from build123d import *

# Parameters (mm, degrees)
SKETCH1_R           = 3.175
BOSS_EXTRUDE1_DEPTH = 1.3843


with BuildPart() as part:
    # Sketch1 → Boss-Extrude1 (new body, symmetric)
    with BuildSketch(Plane.XY):
        with BuildLine():
            Line((-9.281911907, 14.838161907), (-11.983546213, 3.110176509))
            ThreePointArc((-11.983546213, 3.110176509), (-11.495811318, 0.958331313), (-9.508369704, 0))
            Line((-9.508369704, 0), (9.508369704, 0))
            ThreePointArc((9.508369704, 0), (11.495811318, 0.958331313), (11.983546213, 3.110176509))
            Line((11.983546213, 3.110176509), (9.281911907, 14.838161907))
            ThreePointArc((9.281911907, 14.838161907), (0, 22.225), (-9.281911907, 14.838161907))
        make_face()
        with Locations((0, 12.7)):
            Circle(SKETCH1_R, mode=Mode.SUBTRACT)
    extrude(amount=BOSS_EXTRUDE1_DEPTH, both=True)


solid = part.part
Geometry check sheet. Reference: the model listing, model coordinates, mm. Round coordinates to 2 decimals unless told otherwise and drop trailing zeros. Order: outer loops, then holes, each group sorted by start corner. A loop starts at its lowest first (then second) coordinate and runs counter-clockwise, first axis right, second up. Notation, with made-up numbers: M 85,28 L 116,28 A33 cw 116,64 Z; hole C 9,2.5 d8. An arc over 180 degrees is marked long. Answer in a Markdown table with one row per item.
(1) Sectioned sample at A-A, the plane z = -0.9. Record the cut outline in (x, y) (3 decimals).
Responses:
| item | result |
|---|---|
| outline | M -11.984,3.11 A2.54 ccw -9.508,0 L 9.508,0 A2.54 ccw 11.984,3.11 L 9.282,14.838 A9.525 ccw -9.282,14.838 Z; hole C 0,12.7 d6.35 |
(2) Sectioned sample at D-D, the plane x = 5.5. Record the cut outline in (y, z), and give its area (3 significant figures).
Responses:
| item | result |
|---|---|
| outline | M 0,-1.38 L 20.48,-1.38 L 20.48,1.38 L 0,1.38 Z |
| area | 56.7 mm² |
(3) Sectioned sample at C-C, the plane y = 13.75. Record the cut outline in (x, z), and give its area (3 significant figures).
Responses:
| item | result |
|---|---|
| outline | M -9.53,-1.38 L -3,-1.38 L -3,1.38 L -9.53,1.38 Z; M 3,-1.38 L 9.53,-1.38 L 9.53,1.38 L 3,1.38 Z |
| area | 36.2 mm² |
(4) Sectioned sample at B-B, the plane x = 0. Record the cut outline in (y, z) (3 decimals).
Responses:
| item | result |
|---|---|
| outline | M 0,-1.384 L 9.525,-1.384 L 9.525,1.384 L 0,1.384 Z; M 15.875,-1.384 L 22.225,-1.384 L 22.225,1.384 L 15.875,1.384 Z |
(5) Scan lines: probe 1 along Y at (x, z) = (0, -0.7) (3 decimals); probe 2 along X at (y, z) = (13.25, 0.05); probe 3 along Y at (x, z) = (-2, -1.05). Record each from-to range of solid material in increasing order. Write a range as from..to.
Responses:
| item | result |
|---|---|
| probe 1 | y = 0..9.525, 15.875..22.225 |
| probe 2 | x = -9.65..-3.13, 3.13..9.65 |
| probe 3 | y = 0..10.23, 15.17..22.01 |
(6) Draft check along Y on faces 1 (the face through (0, 0, 0)), 2 (the face through (1.5, 9.9, 0)), 3 (the face through (0, 9, -1.384)), 4 (the face through (10.652, 8.892, 0.019)). Enter one of: released by +Y, released by -Y, zero draft, split by the parting line, or undercut.
Responses:
| item | result |
|---|---|
| face 1 | released by -Y |
| face 2 | undercut |
| face 3 | zero draft |
| face 4 | released by +Y |
(7) Go/stop test with flat-tipped pins: P1, Ø1.5, axis at x = -4.5, z = 0.5, coming from the +Y side; P2, Ø1.5, axis at y = 16.5, z = 1, coming from the -X side. Record where each tip stops, or that it passes through.
Responses:
| item | result |
|---|---|
| P1 | stops at y = 21.46 |
| P2 | stops at x = -9.02 |
